from build123d import *

# Parameters (mm, degrees)
SKETCH1_R           = 3
BOSS_EXTRUDE1_DEPTH = 14
SKETCH2_W           = 6
SKETCH2_H           = 12
CUT_EXTRUDE1_DEPTH  = 108.591821251


with BuildPart() as part:
    # Sketch1 → Boss-Extrude1 (new body)
    # profile 1 of 2: a face of its own
    with BuildSketch(Plane(origin=(0, 0, 0), x_dir=(1, 0, 0), z_dir=(0, 1, 0))):
        with BuildLine():
            Line((100, 6), (-10, 6))
            ThreePointArc((-10, 6), (-16, 0), (-10, -6))
            Line((-10, -6), (100, -6))
            ThreePointArc((100, -6), (106, 0), (100, 6))
        make_face()
        with Locations(Location((-10, 0, 0), (0, 0, 90))):
            Circle(SKETCH1_R, mode=Mode.SUBTRACT)
        with BuildLine():
            ThreePointArc((100, -2), (102, 0), (100, 2))
            Line((100, 2), (0, 2))
            ThreePointArc((0, 2), (-2, 0), (0, -2))
            Line((0, -2), (100, -2))
        make_face(mode=Mode.SUBTRACT)
    # profile 2 of 2: a face of its own
    with BuildSketch(Plane(origin=(0, 0, 0), x_dir=(1, 0, 0), z_dir=(0, 1, 0))):
        with BuildLine():
            Line((43.420617055, 2), (35.173899985, 2))
            ThreePointArc((35.173899985, 2), (37.173899985, 0), (35.173899985, -2))
            Line((35.173899985, -2), (43.420617055, -2))
            ThreePointArc((43.420617055, -2), (41.420617055, 0), (43.420617055, 2))
        make_face()
    extrude(amount=BOSS_EXTRUDE1_DEPTH)

    # Sketch2 → Cut-Extrude1 (cut, through all)
    with BuildSketch(Plane.XY.offset(6)):
        with BuildLine():
            Line((-10, 0), (26.424428901, 0))
            ThreePointArc((26.424428901, 0), (25.801654438, 0.065353178), (25.206013503, 0.258565354))
            Line((25.206013503, 0.258565354), (-0.630442404, 11.741434646))
            ThreePointArc((-0.630442404, 11.741434646), (-1.226083339, 11.934646822), (-1.848857802, 12))
            Line((-1.848857802, 12), (-10, 12))
            Line((-10, 12), (-10, 0))
        make_face()
        with BuildLine():
            Line((26.848857802, 2), (100, 2))
            Line((100, 2), (100, 14))
            Line((100, 14), (-1.424428901, 14))
            ThreePointArc((-1.424428901, 14), (-0.801654438, 13.934646822), (-0.206013503, 13.741434646))
            Line((-0.206013503, 13.741434646), (25.630442404, 2.258565354))
            ThreePointArc((25.630442404, 2.258565354), (26.226083339, 2.065353178), (26.848857802, 2))
        make_face()
        with Locations((103, 8)):
            Rectangle(SKETCH2_W, SKETCH2_H)
        with Locations((-13, 6)):
            Rectangle(SKETCH2_W, SKETCH2_H)
    extrude(amount=-CUT_EXTRUDE1_DEPTH, mode=Mode.SUBTRACT)


solid = part.part
For this review, take the finished solid that the model builds, in its own axes (mm). A direction names the side the tool comes from. Round coordinates to 2 decimals unless told otherwise and drop trailing zeros. Order: outer loops, then holes, each group sorted by start corner. A loop starts at its lowest first (then second) coordinate and runs counter-clockwise, first axis right, second up. Notation, with made-up numbers: M 86.5,86 L 143.5,86 A23 ccw 143.5,116 Z; hole C -40,22.5 d3. An arc over 180 degrees is marked long. Write each question's results on one line, items separated by ' | '. Start each with the question number.
1. Add section D-D (x = 40). State the section outline as (y, z) points.
2. Draft analysis for pull direction X (two halves, no side actions). For faces 6 (the face through (102, 1, 0)), 7 (the face through (12.47, 5.92, -3.92)), 8 (the face through (18, 5, -2)), state which applies: pulls with the +X half, pulls with the -X half, needs draft (parallel to the pull), parting line crosses it, or undercut.
3. Add section A-A (x = 98.5). State the section outline as (y, z) points.
4. To check wall thickness, follow L1, parallel to X at y = 12.6, z = 0; L2, parallel to Z at x = -10, y = 13.4; L3, parallel to Y at x = 40, z = 5.5. State the ranges of each line that lie inside material, in increasing order. Write a range as [from, to].
5. Add section B-B (y = 7.25). State the section outline as (x, z) points.
6. Add section C-C (z = 4). State the section outline as (x, y) points.
7. Clearance check with flat-ended pins moving along their axes: pin 1 Ø5 at (x, z) = (47.5, 0.5) entering from +Y; pin 2 Ø4 at (y, z) = (9.5, -2) entering from -X; pin 3 Ø4 at (x, z) = (9, -1) entering from -Y. State where each tip first meets the part, or that it passes through.
8. Tool access review of faces 1 (the face through (71, 1, 2)), 2 (the face through (66, 0, -3)), 3 (the face through (66, 2, 3)), 4 (the face through (-7, 12, 1)), 5 (the face through (-2, 13, 0)): name each direction out of +Z, -Z, +X, -X, +Y, -Y from which nothing blocks a thin tool from reaching the whole face with its end or side.
Output values:
1) outline: M 0,-6 L 2,-6 L 2,6 L 0,6 Z
2) face 6: undercut | face 7: pulls with the -X half | face 8: needs draft
3) outline: M 0,-6 L 2,-6 L 2,-2 L 0,-2 Z; M 0,2 L 2,2 L 2,6 L 0,6 Z
4) L1: [-16, -13], [-7, -2] | L2: [-6, -3], [3, 6] | L3: [0, 2]
5) outline: M 9.48,-6 L 14.4,-6 L 14.4,-2 L 9.48,-2 Z; M 9.48,2 L 14.4,2 L 14.4,6 L 9.48,6 Z
6) outline: M -14.47,12 L -1.85,12 A3 cw -0.63,11.74 L 25.21,0.26 A3 ccw 26.42,0 L 104.47,0 L 104.47,2 L 26.85,2 A3 cw 25.63,2.26 L -0.21,13.74 A3 ccw -1.42,14 L -14.47,14 Z
7) pin 1: y = 2 | pin 2: x = -0.09 | pin 3: y = 6.69
8) face 1: +Y, -Y | face 2: +Z, -Z, +X, -X, -Y | face 3: +Z, -Z, +X, +Y | face 4: +Z, -Z, -X, -Y | face 5: +X, +Y, -Y
